Geometry: final body of the model. Coordinates: model frame, mm. A direction names the side the tool comes from. Coordinates: 2 decimals unless noted, no trailing zeros. Order: outer loops, then holes, each group sorted by start corner. A loop starts at its lowest first (then second) coordinate and runs counter-clockwise, first axis right, second up. Notation, with made-up numbers: M 46,-12 L 100,-12 A24 ccw 100,19 Z; hole C -20.75,38 d11. An arc over 180 degrees is marked long. Write item = value, one per line. Start each with the question number.
```python
from build123d import *

# Parameters (mm, degrees)
F0_W     = 140
F0_H     = 70
F1_DEPTH = 60
F2_W     = 30
F2_H     = 30
F3_DEPTH = 60
F4_W     = 30
F4_H     = 30
F5_DEPTH = 60


with BuildPart() as f1:
    # F0 (on Front) → F1 (new body)
    with BuildSketch(Plane.XZ):
        with Locations((7.357027, 12.952588)):
            Rectangle(F0_W, F0_H)
    extrude(amount=F1_DEPTH)

    # F2 (on face) → F3 (cut)
    with BuildSketch(Plane(origin=(0, 0, -22.047412), x_dir=(1, 0, 0), z_dir=(0, 0, -1))):
        with Locations((-47.642973, 45)):
            Rectangle(F2_W, F2_H)
    extrude(amount=-F3_DEPTH, mode=Mode.SUBTRACT)

    # F4 (on face) → F5 (cut)
    with BuildSketch(Plane(origin=(0, 0, -22.047412), x_dir=(1, 0, 0), z_dir=(0, 0, -1))):
        with Locations((62.357027, 45)):
            Rectangle(F4_W, F4_H)
    extrude(amount=-F5_DEPTH, mode=Mode.SUBTRACT)


solid = f1.part
```
Item 1: Section query A-A on y = -48.5. Output: boundary loops of the cut face in (x, z).
Item 2: Reachability of faces 1 (the flat face through (6, -23, -22.047)), 2 (the flat face through (-32.643, -45, 8)), 3 (the flat face through (62, -30, 8)) from +Z, -Z, +X, -X, +Y, -Y: full face, straight path, thin tool, end or side. Return the list, or none.
Item 3: Section query B-B on z = 23. Output: boundary loops of the cut face in (x, y).
Item 4: First-contact query: pin 1 (6 mm diameter, centred on x = 25.5, z = 5.5, fed in from +Y); pin 2 (24 mm diameter, centred on x = 60, z = 7.5, fed in from -Y); pin 3 (9 mm diameter, centred on y = -39, z = 2, fed in from -X); pin 4 (9 mm diameter, centred on y = -50, z = -0.5, fed in from +X). Flat tips, straight axial feed; report the tip coordinate or a pass-through.
Item 5: Section query C-C on x = 65. Output: boundary loops of the cut face in (y, z).
Item 6: Material intervals for probe 1 along X at (y, z) = (-40, 17.5); probe 2 along Y at (x, z) = (-51, 35); probe 3 along Z at (x, y) = (-54, -36), sorted ascending. Write a range as [from, to].
Ans:
q1.outline = M -62.64,37.95 L -32.64,37.95 L -32.64,-22.05 L 47.36,-22.05 L 47.36,37.95 L 77.36,37.95 L 77.36,47.95 L -62.64,47.95 Z
q2.face_1 = -Z, +X, -X, +Y, -Y
q2.face_2 = -Z, -X, -Y
q2.face_3 = -Z, +X, -Y
q3.outline = M -62.64,-30 L -32.64,-30 L -32.64,-60 L 47.36,-60 L 47.36,-30 L 77.36,-30 L 77.36,0 L -62.64,0 Z
q4.pin_1 = 0
q4.pin_2 = -30
q4.pin_3 = -32.64
q4.pin_4 = 47.36
q5.outline = M -60,37.95 L -30,37.95 L -30,-22.05 L 0,-22.05 L 0,47.95 L -60,47.95 Z
q6.probe_1 = [-32.64, 47.36]
q6.probe_2 = [-30, 0]
q6.probe_3 = [37.95, 47.95]
